Part model, mm, in its own coordinate system. Face numbers are marked on the shaded views. Round coordinates to 2 decimals unless told otherwise and drop trailing zeros. Use a Markdown table: item, result. Add a question column.
1) Two-plate mould, pull along Y, no slides. Class the marked faces 1, 2 and 3: released by +Y, released by -Y, zero draft, split by the parting line, or undercut.
2) Wall check: probe 1 along Y at (x, z) = (0, -3.3) (1 decimal); probe 2 along X at (y, z) = (2.75, -3.15); probe 3 along X at (y, z) = (-2, -4.5). Give the ranges that are in metal, low to high.
3) Drop a flat-ended pin along its axis: P1, Ø1, axis at x = 4, y = 4.5, coming from the +Z side. Give the stop position or say it passes through.
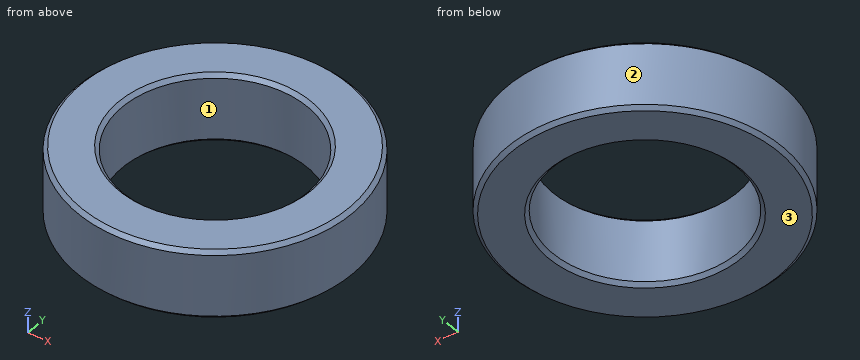
Autodesk Inventor part; units mm, degrees
ref_plane "YZ Plane" through (0, 0, 0) normal (1, 0, 0) x (0, 1, 0)
ref_plane "XZ Plane" through (0, 0, 0) normal (0, 1, 0) x (-1, 0, 0)
ref_plane "XY Plane" through (0, 0, 0) normal (0, 0, 1) x (1, 0, 0)
sketch "Sketch1" plane through (0, 0, 0) normal (0, 0, 1) x (1, 0, 0)
  circle A0 centre (0, 0) radius 6.4135
  circle A1 centre (0, 0) radius 9.525
  dimension "d0" = 12.827
  dimension "d1" = 19.05
extrude "Extrusion1" add sketch "Sketch1" against normal blind 4.7752
chamfer "Chamfer1" distance 0.254 angle 45 4 edges at (-9.525, 0, 0) (-6.4135, 0, 0) (-9.525, 0, -4.7752) (-6.4135, 0, -4.7752)
properties part number "am-2271" material "Nylon-6/6"
Entries:
| question | item | result |
|---|---|---|
| 1 | face 1 | undercut |
| 1 | face 2 | split by the parting line |
| 1 | face 3 | zero draft |
| 2 | probe 1 | y = -9.5 to -6.4, 6.4 to 9.5 |
| 2 | probe 2 | x = -9.12 to -5.79, 5.79 to 9.12 |
| 2 | probe 3 | x = -9.31 to -6.09, 6.09 to 9.31 |
| 3 | P1 | stops at z = -0.15 |
